Autodesk Inventor part; units mm, degrees
ref_plane "1_XY" through (0, 0, -7.5) normal (0, 0, 1) x (1, 0, 0)
ref_plane "1_YZ" through (0, 0, -7.5) normal (1, 0, 0) x (0, 1, 0)
ref_plane "1_ZX" through (0, 0, -7.5) normal (0, 1, 0) x (0, 0, 1)
sketch "Sketch_1" plane through (0, 0, 0) normal (1, 0, 0) x (0, 1, 0)
  line L0 (0, -7.5) -> (0, 7.5)
  line L1 (4.6, 7.5) -> (4.6, -7.5)
  line L2 (4.6, -7.5) -> (12, -7.5)
  line L3 (12, -7.5) -> (12, -2.5)
  line L4 (12, -2.5) -> (14.5, -2.5)
  line L5 (14.5, -2.5) -> (14.5, 3.5)
  line L6 (14.5, 3.5) -> (12, 3.5)
  line L7 (12, 3.5) -> (12, 7.5)
  line L8 (12, 7.5) -> (4.6, 7.5)
revolve "Revolution1" add sketch "Sketch_1" angle 360 about axis through (0, 0, -7.5) along (0, 0, -1)
ref_plane "1_XY" through (0, 0, -7.5) normal (0, 0, 1) x (1, 0, 0)
ref_plane "1_YZ" through (0, 0, -7.5) normal (1, 0, 0) x (0, 1, 0)
ref_plane "1_ZX" through (0, 0, -7.5) normal (0, 1, 0) x (0, 0, 1)
ref_plane "2_XY" through (0, 0, 7.5) normal (0, 0, 1) x (1, 0, 0)
ref_plane "2_YZ" through (0, 0, 7.5) normal (1, 0, 0) x (0, 1, 0)
ref_plane "2_ZX" through (0, 0, 7.5) normal (0, 1, 0) x (0, 0, 1)
properties part number "HFROLL5_b"
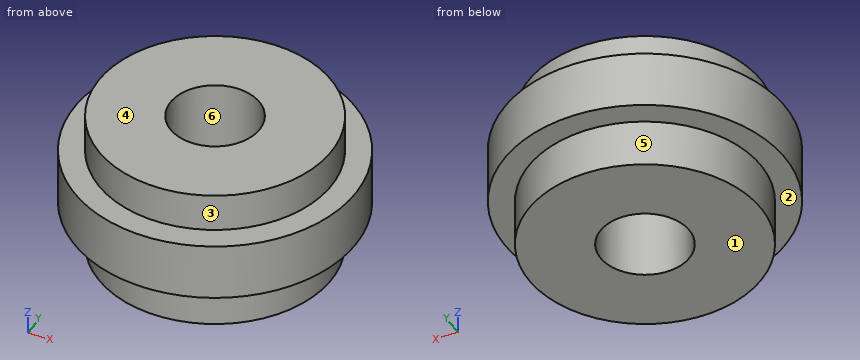
For this review, take the finished solid that the model builds, in its own axes (mm). Face numbers are marked on the shaded views. A direction names the side the tool comes from. Round coordinates to 2 decimals unless told otherwise and drop trailing zeros. Loops run counter-clockwise (first coordinate to the right, second up) from the corner with the lowest first, then second, coordinate; pieces in that order, holes last.
(1) We need section D-D (x = -6.5). Give the boundary of the cut face in (y, z).
Returned:
outline: (-12.96, -2.5) - (-10.09, -2.5) - (-10.09, -7.5) - (10.09, -7.5) - (10.09, -2.5) - (12.96, -2.5) - (12.96, 3.5) - (10.09, 3.5) - (10.09, 7.5) - (-10.09, 7.5) - (-10.09, 3.5) - (-12.96, 3.5) - close
(2) We need section A-A (x = 0). Give the boundary of the cut face in (y, z), plus the area to 3 significant figures.
Returned:
outline: (-14.5, -2.5) - (-12, -2.5) - (-12, -7.5) - (-4.6, -7.5) - (-4.6, 7.5) - (-12, 7.5) - (-12, 3.5) - (-14.5, 3.5) - close; (4.6, -7.5) - (12, -7.5) - (12, -2.5) - (14.5, -2.5) - (14.5, 3.5) - (12, 3.5) - (12, 7.5) - (4.6, 7.5) - close
area: 252 mm2
(3) We need section C-C (z = 1). Give the boundary of the cut face in (x, y), plus the area to 3 significant figures.
Returned:
outline: circle Ø29 at (0, 0); hole circle Ø9.2 at (0, 0)
area: 594 mm2
(4) Wall thickness on line 1 along X through (y, z) = (0, -1.5); line 2 along X through (y, z) = (0, -4); line 3 along Z through (x, y) = (11, 8.25): over which ranges is each line inside the solid? List them lowest first.
Returned:
line 1: x = -14.5 to -4.6, 4.6 to 14.5
line 2: x = -12 to -4.6, 4.6 to 12
line 3: z = -2.5 to 3.5
(5) Tool access review of the marked faces 1, 2 and 3: name each direction out of +Z, -Z, +X, -X, +Y, -Y from which nothing blocks a thin tool from reaching the whole face with its end or side.
Returned:
face 1: -Z, +X, -X, +Y, -Y
face 2: -Z
face 3: +Z
(6) Clearance check with flat-ended pins moving along their axes: P1, Ø12, axis at x = 0, y = 0, coming from the +Z side; P2, Ø1, axis at x = 2, z = -2.5, coming from the -Y side; P3, Ø5, axis at y = -8, z = -1.5, coming from the -X side; P4, Ø5, axis at y = 10.5, z = 3, coming from the +X side. State where each tip first meets the part, or that it passes through.
Returned:
P1: stops at z = 7.5
P2: stops at y = -14.42
P3: stops at x = -13.42
P4: stops at x = 12.09
(7) Mouldability with a two-part tool opening along X and no side actions: class the marked faces 4, 5 and 6 as released by +X, released by -X, zero draft, split by the parting line, or undercut.
Returned:
face 4: zero draft
face 5: split by the parting line
face 6: undercut
